Read the model definition and answer for the solid it produces. Units are mm, in the model's axes. Give positions to 0.01 mm unless a question says otherwise; leave off trailing zeros. Order: outer loops, then holes, each group sorted by start corner. A loop starts at its lowest first (then second) coordinate and runs counter-clockwise, first axis right, second up. Notation, with made-up numbers: (-26, 58) - (-12, 58) arc R18 ccw to (-12, 74) - close; hole circle Ø11 at (36, -11.75). An arc over 180 degrees is marked (long way). Return JSON: item names as keys, results as strings.
```python
from build123d import *

# Parameters (mm, degrees)
MODEL_R                 = 1.6
MODEL_R_2               = 2.75
MODEL_W                 = 5.5
MODEL_H                 = 5
SALIENTE_EXTRUIR1_DEPTH = 3


with BuildPart() as part:
    # Model → Saliente-Extruir1 (new body)
    with BuildSketch(Plane.XY):
        with BuildLine():
            Line((136.131313967, 8.172644832), (28.691078747, 8.175075185))
            ThreePointArc((28.691078747, 8.175075185), (28.098964944, 7.980929542), (27.736763771, 7.473877674))
            Line((27.736763771, 7.473877674), (26.175859161, 2.488662696))
            ThreePointArc((26.175859161, 2.488662696), (25.813657989, 1.981610828), (25.221544186, 1.787465185))
            Line((25.221544186, 1.787465185), (5.956313823, 1.787465185))
            ThreePointArc((5.956313823, 1.787465185), (2.420778394, 3.251930446), (0.956311467, 6.787465185))
            Line((0.956311467, 6.787465185), (0.956311467, 41.175060185))
            ThreePointArc((0.956311467, 41.175060185), (2.420777561, 44.710594091), (5.956311467, 46.175060185))
            Line((5.956311467, 46.175060185), (10.956311467, 46.175060185))
            Line((10.956311467, 46.175060185), (40.628815467, 46.175060185))
            ThreePointArc((40.628815467, 46.175060185), (40.982368857, 46.321506794), (41.128815467, 46.675060185))
            Line((41.128815467, 46.675060185), (41.128815467, 52.173080185))
            ThreePointArc((41.128815467, 52.173080185), (41.714601904, 53.587293747), (43.128815467, 54.173080185))
            Line((43.128815467, 54.173080185), (47.444968064, 54.173080185))
            ThreePointArc((47.444968064, 54.173080185), (47.886694472, 53.907340256), (47.858883503, 53.392591309))
            ThreePointArc((47.858883503, 53.392591309), (51.128815467, 47.226729185), (54.39874743, 53.392591309))
            ThreePointArc((54.39874743, 53.392591309), (54.370936461, 53.907340256), (54.812662869, 54.173080185))
            Line((54.812662869, 54.173080185), (59.128815467, 54.173080185))
            ThreePointArc((59.128815467, 54.173080185), (60.543029029, 53.587293747), (61.128815467, 52.173080185))
            Line((61.128815467, 52.173080185), (61.128815467, 46.675057185))
            ThreePointArc((61.128815467, 46.675057185), (61.275262076, 46.321503794), (61.628815467, 46.175057185))
            Line((61.628815467, 46.175057185), (136.131313967, 46.175058685))
            Line((136.131313967, 46.175058685), (210.633812467, 46.175057185))
            ThreePointArc((210.633812467, 46.175057185), (210.987365857, 46.321503794), (211.133812467, 46.675057185))
            Line((211.133812467, 46.675057185), (211.133812467, 52.173080185))
            ThreePointArc((211.133812467, 52.173080185), (211.719598904, 53.587293747), (213.133812467, 54.173080185))
            Line((213.133812467, 54.173080185), (217.449965065, 54.173080185))
            ThreePointArc((217.449965065, 54.173080185), (217.891691472, 53.907340256), (217.863880503, 53.392591309))
            ThreePointArc((217.863880503, 53.392591309), (221.133812467, 47.226729185), (224.403744431, 53.392591309))
            ThreePointArc((224.403744431, 53.392591309), (224.375933462, 53.907340256), (224.81765987, 54.173080185))
            Line((224.81765987, 54.173080185), (229.133812467, 54.173080185))
            ThreePointArc((229.133812467, 54.173080185), (230.548026029, 53.587293747), (231.133812467, 52.173080185))
            Line((231.133812467, 52.173080185), (231.133812467, 46.675060185))
            ThreePointArc((231.133812467, 46.675060185), (231.280259076, 46.321506794), (231.633812467, 46.175060185))
            Line((231.633812467, 46.175060185), (261.306316467, 46.175060185))
            Line((261.306316467, 46.175060185), (266.306316467, 46.175060185))
            ThreePointArc((266.306316467, 46.175060185), (269.841850373, 44.710594091), (271.306316467, 41.175060185))
            Line((271.306316467, 41.175060185), (271.306316467, 6.787465185))
            ThreePointArc((271.306316467, 6.787465185), (269.84184954, 3.251930446), (266.306314111, 1.787465185))
            Line((266.306314111, 1.787465185), (247.041083748, 1.787465185))
            ThreePointArc((247.041083748, 1.787465185), (246.448969945, 1.981610828), (246.086768772, 2.488662696))
            Line((246.086768772, 2.488662696), (244.525864162, 7.473877674))
            ThreePointArc((244.525864162, 7.473877674), (244.16366299, 7.980929542), (243.571549187, 8.175075185))
            Line((243.571549187, 8.175075185), (136.131313967, 8.172644832))
        make_face()
        with Locations((51.128815467, 36.176729185)):
            Circle(MODEL_R, mode=Mode.SUBTRACT)
        with Locations((221.133812467, 36.176729185)):
            Circle(MODEL_R, mode=Mode.SUBTRACT)
        with Locations((143.631313967, 27.173851758)):
            Circle(MODEL_R, mode=Mode.SUBTRACT)
        with Locations((23.017213967, 18.787465185)):
            Circle(MODEL_R_2, mode=Mode.SUBTRACT)
        with Locations((249.575379967, 18.787465185)):
            Circle(MODEL_R_2, mode=Mode.SUBTRACT)
        with Locations((143.631313967, 34.673851758)):
            Rectangle(MODEL_W, MODEL_H, mode=Mode.SUBTRACT)
        with Locations((143.631313967, 19.673851758)):
            Rectangle(MODEL_W, MODEL_H, mode=Mode.SUBTRACT)
    extrude(amount=SALIENTE_EXTRUIR1_DEPTH)


solid = part.part
```
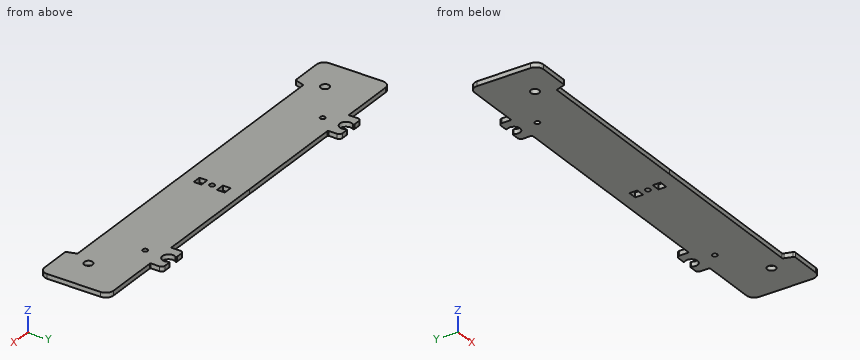
Q1. A cutting plane is placed at A-A (x = 164). Write down the section's boundary in (y, z).
Values:
{"outline": "(8.17, 0) - (46.18, 0) - (46.18, 3) - (8.17, 3) - close"}
Q2. Consider L1, parallel to X at y = 19, z = 1.85; L2, parallel to X at y = 49.5, z = 1.95; L3, parallel to X at y = 7.5, z = 1.85. Determine where each line is inside the solid, lowest interval first.
Values:
{"L1": "x = 0.96 to 20.28, 25.76 to 140.88, 146.38 to 246.83, 252.32 to 271.31", "L2": "x = 41.13 to 47.55, 54.71 to 61.13, 211.13 to 217.56, 224.71 to 231.13", "L3": "x = 0.96 to 27.75, 244.52 to 271.31"}
Q3. Given pin 1 (0.9 mm diameter, centred on x = 249, z = 1, fed in from +Y); pin 2 (1.5 mm diameter, centred on x = 143.5, z = 1.5, fed in from -Y), each flat-ended and moving along its own axis, determine where each tip first touches the part or whether it passes through.
Values:
{"pin 1": "stops at y = 46.18", "pin 2": "stops at y = 8.17"}
Q4. A cutting plane is placed at B-B (z = 0.65). Give the number of separate pieces and of enclosed holes in the cut face, and give its area (3 significant figures).
Values:
{"separate pieces": "1", "enclosed holes": "7", "area": "10,700 mm²"}
